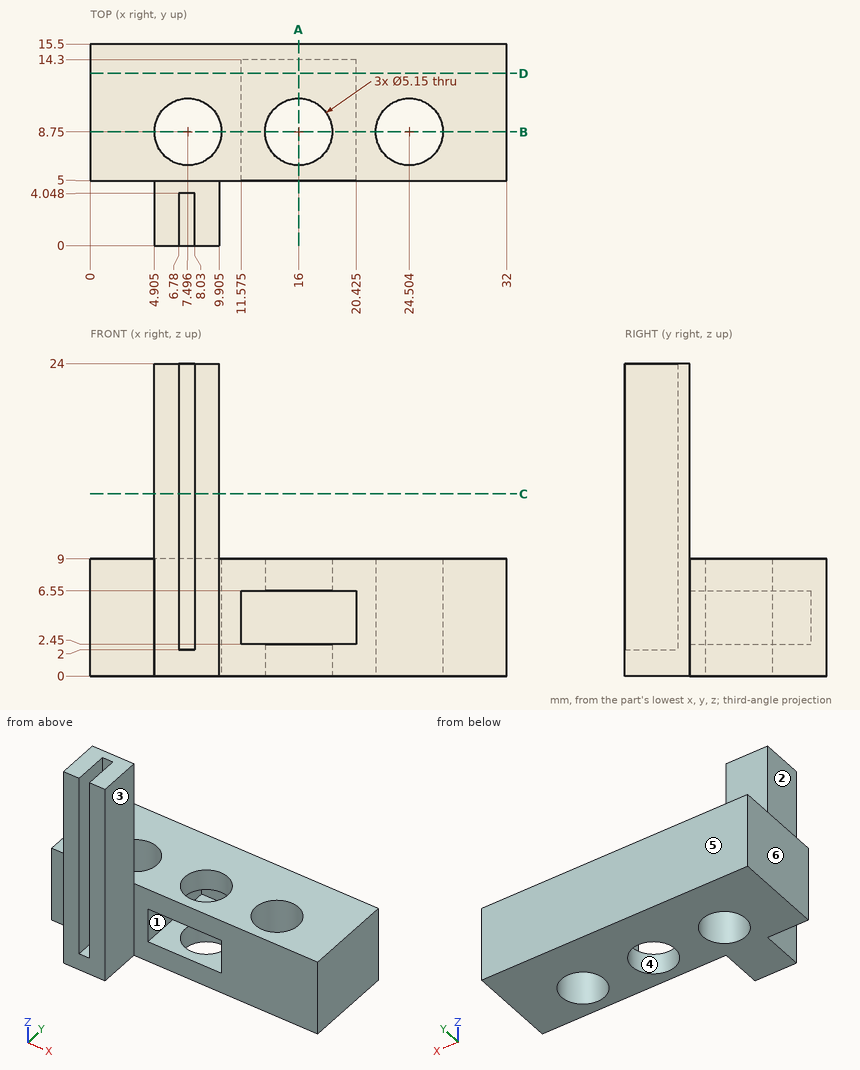
The figure shows three views and two pictorial views of one solid part (mm, origin at its lowest corner). Answer the questions. A direction names the side the tool comes from. Give positions to 0.01 mm unless a question says otherwise; leave off trailing zeros. Loops run counter-clockwise (first coordinate to the right, second up) from the corner with the lowest first, then second, coordinate; pieces in that order, holes last. Notation, with made-up numbers: (2.5, -30) -> (52.5, -30) arc R30 ccw to (52.5, 2) -> close; hole circle Ø4 at (49.25, 9.5). An arc over 180 degrees is marked (long way). Put each result on its own line as item: value. Start each with the question number.
Item 1: Each of these flat-tipped pins is pushed along its axis until it touches: P1, Ø4, axis at y = 6, z = 19.5, coming from the -X side (3 decimals); P2, Ø4, axis at y = 2.5, z = 13, coming from the +X side (3 decimals); P3, Ø3, axis at x = 9, y = 11.5, coming from the +Z side. Where does it stop, or does it pass through?
Item 2: The part is cut by section C-C (z = 14). Give the vertices of the cut face in (x, y) (3 decimals), then the cut area to 3 significant figures.
Item 3: Which of the six approach directions +Z, -Z, +X, -X, +Y, -Y give full straight-line access (tool end or side, diameter ignored) to the marked faces 1, 2 and 3?
Item 4: The part is cut by section A-A (x = 16). Give the vertices of the cut face in (y, z) (3 decimals).
Item 5: Find the intervals of material crossed by L1, parallel to X at y = 8.75, z = 6.75 (3 decimals); L2, parallel to Z at x = 20, y = 7; L3, parallel to X at y = 3, z = 19.5 (3 decimals), in increasing order. Write a range as [from, to].
Item 6: The part is cut by section B-B (y = 8.75). Give the vertices of the cut face in (x, z) (3 decimals), then the cut area to 3 significant figures.
Item 7: The mould has two halves that part along X. Classify the marked faces 4, 5 and 6: released by +X, released by -X, zero draft, split by the parting line, or undercut.
Item 8: The part is cut by section D-D (y = 13.25). Give the vertices of the cut face in (x, z) (3 decimals).
Answers below:
1. P1: x = 4.905
1. P2: x = 9.905
1. P3: z = 9
2. outline: (4.905, 0) -> (6.78, 0) -> (6.78, 4.048) -> (8.03, 4.048) -> (8.03, 0) -> (9.905, 0) -> (9.905, 5) -> (4.905, 5) -> close
2. area: 19.9 mm2
3. face 1: -Y
3. face 2: +Z, -Z, -X, -Y
3. face 3: +Z, -Z, +X, -Y
4. outline: (5, 0) -> (6.175, 0) -> (6.175, 2.45) -> (5, 2.45) -> close; (5, 6.55) -> (6.175, 6.55) -> (6.175, 9) -> (5, 9) -> close; (11.325, 0) -> (15.5, 0) -> (15.5, 9) -> (11.325, 9) -> (11.325, 6.55) -> (14.3, 6.55) -> (14.3, 2.45) -> (11.325, 2.45) -> close
5. L1: [0, 4.921], [10.071, 13.425], [18.575, 21.929], [27.079, 32]
5. L2: [0, 2.45], [6.55, 9]
5. L3: [4.905, 6.78], [8.03, 9.905]
6. outline: (0, 0) -> (4.921, 0) -> (4.921, 9) -> (0, 9) -> close; (10.071, 0) -> (13.425, 0) -> (13.425, 2.45) -> (11.575, 2.45) -> (11.575, 6.55) -> (13.425, 6.55) -> (13.425, 9) -> (10.071, 9) -> close; (18.575, 0) -> (21.929, 0) -> (21.929, 9) -> (18.575, 9) -> (18.575, 6.55) -> (20.425, 6.55) -> (20.425, 2.45) -> (18.575, 2.45) -> close; (27.079, 0) -> (32, 0) -> (32, 9) -> (27.079, 9) -> close
6. area: 134 mm2
7. face 4: undercut
7. face 5: zero draft
7. face 6: released by -X
8. outline: (0, 0) -> (32, 0) -> (32, 9) -> (0, 9) -> close; hole (11.575, 2.45) -> (20.425, 2.45) -> (20.425, 6.55) -> (11.575, 6.55) -> close
